CAD build for the part. Positions are in the model's coordinates, mm. A direction names the side the tool comes from. Give positions to 0.01 mm unless a question says otherwise; leave off trailing zeros. Order: outer loops, then holes, each group sorted by start corner. A loop starts at its lowest first (then second) coordinate and runs counter-clockwise, first axis right, second up.
```python
from build123d import *

# Parameters (mm, degrees)
SKETCH008_W  = 26
SKETCH008_H  = 33
PAD002_DEPTH = 17
SKETCH009_R  = 5
PAD003_DEPTH = 34
SKETCH011_R  = 9.75
PAD004_DEPTH = 1.5
FILLET002_R  = 1
FILLET003_R  = 1


with BuildPart() as part:
    # Sketch008 → Pad002 (new body)
    with BuildSketch(Plane.XY):
        with Locations((13, 16.5)):
            Rectangle(SKETCH008_W, SKETCH008_H)
    extrude(amount=PAD002_DEPTH)

    # Sketch009 → Pad003 (join)
    with BuildSketch(Plane.XY):
        with Locations((13, 16.5)):
            Circle(SKETCH009_R)
    extrude(amount=PAD003_DEPTH)

    # Sketch010 → Revolution (revolve)
    with BuildSketch(Plane(origin=(13, 16.5, 2), x_dir=(1, 0, 0), z_dir=(0, -1, 0))):
        with BuildLine():
            Line((0, 24), (0, 17))
            Line((0, 17), (-13, 17))
            ThreePointArc((0, 24), (-7.382412, 22.138764), (-13, 17))
        make_face()
    revolve(axis=Axis((13, 16.5, 2), (0, 0, 1)))

    # Sketch011 → Pad004 (join, symmetric)
    with BuildSketch(Plane.XY.offset(33.5)):
        with Locations((13, 16.5)):
            Circle(SKETCH011_R)
    extrude(amount=PAD004_DEPTH, both=True)

    # Fillet002
    fillet002_edges = [part.edges().sort_by_distance(p)[0] for p in [
        (3.25, 16.5, 35),
    ]]
    fillet(fillet002_edges, radius=FILLET002_R)

    # Fillet003
    fillet003_edges = [part.edges().sort_by_distance(p)[0] for p in [
        (3.25, 16.5, 32),
    ]]
    fillet(fillet003_edges, radius=FILLET003_R)


solid = part.part
```
Item 1: Slice it at C-C (z = 26). Give the cut face in (x, y).
Item 2: Wall check: L1, parallel to Z at x = 19.75, y = 22.5; L2, parallel to Z at x = 10, y = 6; L3, parallel to Z at x = 5, y = 16.5. Give the ranges that are in metal, low to high.
Item 3: Slice it at A-A (x = 2.5). Give the cut face in (y, z).
Item 4: Slice it at B-B (y = 16.5). Give the cut face in (x, z).
Item 5: Drop flat-ended pins along their axis: pin 1 Ø12 at (y, z) = (21.5, 26.5) entering from -X; pin 2 Ø1.5 at (x, z) = (12, 25) entering from +Y; pin 3 Ø4 at (x, z) = (8, 28.5) entering from -Y. Give the stop position or say it passes through.
Item 6: Two-plate mould, pull along Z, no slides. Class faces 4 (the face through (15.307, 12.064, 28.54)), 5 (the face through (13, 17, 35)), 6 (the face through (0, 16, 8)): released by +Z, released by -Z, zero draft, split by the parting line, or undercut.
Item 7: Slice it at D-D (x = 13). Give the cut face in (y, z).
Item 8: Tool access for faces 1 (the face through (15.307, 12.064, 17.986)), 2 (the face through (10.89, 6.98, 33.51)), 3 (the face through (13, 33, 8)): list every direction of +Z, -Z, +X, -X, +Y, -Y with a clear straight run to the whole face (end or side of a thin tool).
A:
1. outline: circle Ø10 at (13, 16.5)
2. L1: z = 0 to 17, 19 to 23.11, 32.04 to 34.96
2. L2: z = 0 to 17, 19 to 21.53
2. L3: z = 0 to 17, 19 to 23.79, 32 to 35
3. outline: (0, 0) - (33, 0) - (33, 17) - (0, 17) - close; (8.84, 19) - (24.16, 19) arc R11.5 ccw to start
4. outline: (0, 0) - (26, 0) - (26, 17) - (18, 17) - (18, 19) - (26, 19) arc R15.57 ccw to (18, 25.18) - (18, 32) - (21.75, 32) arc R1 ccw to (22.75, 33) - (22.75, 34) arc R1 ccw to (21.75, 35) - (4.25, 35) arc R1 ccw to (3.25, 34) - (3.25, 33) arc R1 ccw to (4.25, 32) - (8, 32) - (8, 25.18) arc R15.57 ccw to (0, 19) - (8, 19) - (8, 17) - (0, 17) - close
5. pin 1: stops at x = 1.81
5. pin 2: stops at y = 23.61
5. pin 3: stops at y = 12.5
6. face 4: undercut
6. face 5: released by +Z
6. face 6: zero draft
7. outline: (0, 0) - (33, 0) - (33, 17) - (21.5, 17) - (21.5, 19) - (29.5, 19) arc R15.57 ccw to (21.5, 25.18) - (21.5, 32) - (25.25, 32) arc R1 ccw to (26.25, 33) - (26.25, 34) arc R1 ccw to (25.25, 35) - (7.75, 35) arc R1 ccw to (6.75, 34) - (6.75, 33) arc R1 ccw to (7.75, 32) - (11.5, 32) - (11.5, 25.18) arc R15.57 ccw to (3.5, 19) - (11.5, 19) - (11.5, 17) - (0, 17) - close
8. face 1: none
8. face 2: +Z
8. face 3: +Z, -Z, +X, -X, +Y
